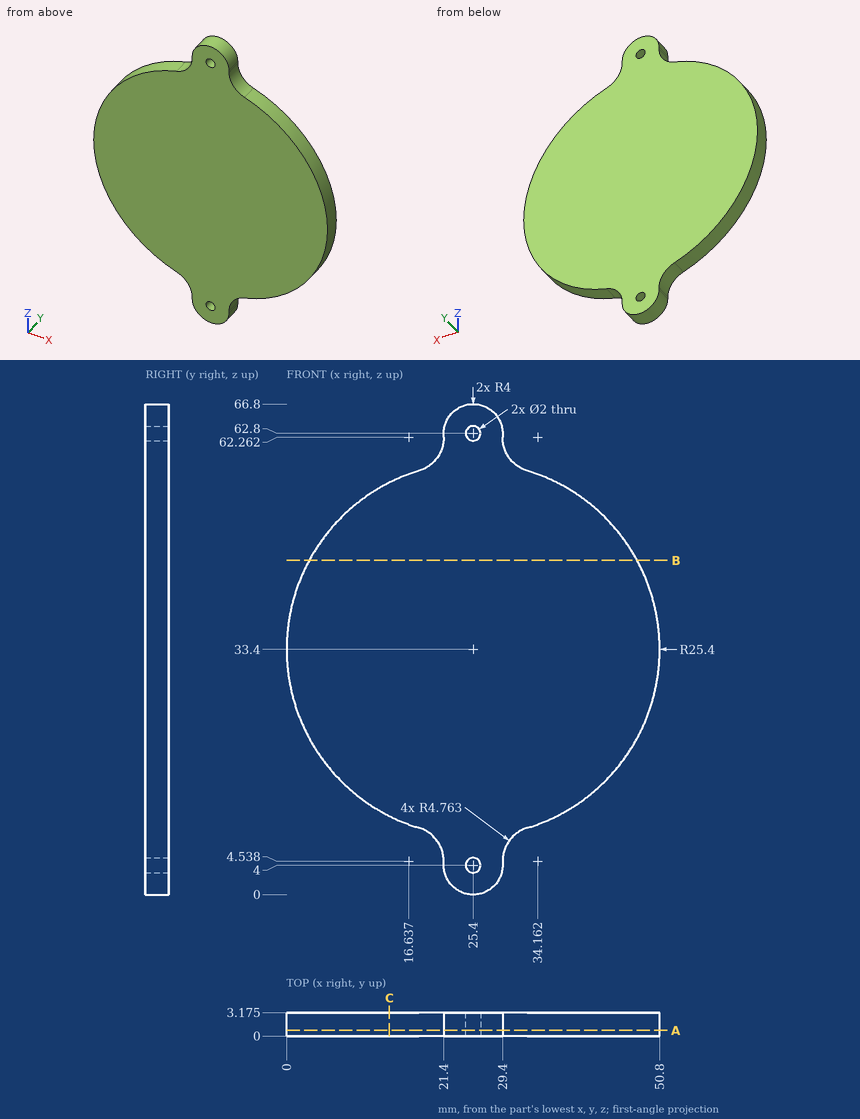
Drawing for the job (mm, zero at the part's lowest x, y, z). Round coordinates to 2 decimals unless told otherwise and drop trailing zeros. Loops run counter-clockwise (first coordinate to the right, second up) from the corner with the lowest first, then second, coordinate; pieces in that order, holes last. Notation, with made-up numbers: (42, 37) - (91, 37) arc R22 ccw to (91, 69) - close; hole circle Ø10 at (87, 4). An arc over 180 degrees is marked (long way). Write each question's results on one line, items separated by ' | '.
(1) Wall check: L1, parallel to Z at x = 25.4, y = 0.9; L2, parallel to X at y = 2.6, z = 63.5 (1 decimal); L3, parallel to X at y = 1, z = 5.5. Give the ranges that are in metal, low to high.
Answer below:
L1: z = 0 to 3, 5 to 61.8, 63.8 to 66.8 | L2: x = 21.5 to 24.7, 26.1 to 29.3 | L3: x = 21.3 to 29.5
(2) Pin check, flat tips, straight feed: pin 1 (1.6 mm diameter, centred on x = 25.4, z = 62.8, fed in from +Y); pin 2 (1 mm diameter, centred on y = 2, z = 20, fed in from -X); pin 3 (0.6 mm diameter, centred on y = 1.5, z = 62.5, fed in from -X). Stop position of each tip, or through.
Answer below:
pin 1: passes through | pin 2: stops at x = 3.52 | pin 3: stops at x = 21.4
(3) Saw through at B-B, the plane z = 45.5. List the corners of the cut face in (x, y) (1 decimal), then the cut area to 3 significant figures.
Answer below:
outline: (3.1, 0) - (47.7, 0) - (47.7, 3.2) - (3.1, 3.2) - close | area: 142 mm^2
(4) Saw through at A-A, the plane y = 0.75. List the corners of the cut face in (x, z) (1 decimal).
Answer below:
outline: (18, 9.1) arc R4.8 cw to (21.4, 4.5) - (21.4, 4) arc R4 ccw to (29.4, 4) - (29.4, 4.5) arc R4.8 cw to (32.8, 9.1) arc R25.4 ccw to (32.8, 57.7) arc R4.8 cw to (29.4, 62.3) - (29.4, 62.8) arc R4 ccw to (21.4, 62.8) - (21.4, 62.3) arc R4.8 cw to (18, 57.7) arc R25.4 ccw to start; hole circle Ø2 at (25.4, 4); hole circle Ø2 at (25.4, 62.8)
(5) Saw through at C-C, the plane x = 14. List the corners of the cut face in (y, z) (1 decimal).
Answer below:
outline: (0, 10.7) - (3.2, 10.7) - (3.2, 56.1) - (0, 56.1) - close
